from build123d import *

# Parameters (mm, degrees)
F0_R     = 12.5
F2_DEPTH = 10
F3_R     = 6.5
F4_DEPTH = 10
F1_R     = 6.5
F5_DEPTH = 10
F7_DEPTH = 10


with BuildPart() as f2:
    # F0 (on Top) → F2 (new body)
    with BuildSketch(Plane.XY):
        Circle(F0_R)
    extrude(amount=F2_DEPTH)

    # F3 (on Top) → F4 (join)
    with BuildSketch(Plane.XY):
        with BuildLine():
            Line((34.328218, 24.012301), (2.916428, 13.975679))
            Line((2.916428, 13.975679), (5.668561, 29.53591))
            ThreePointArc((5.668561, 29.53591), (7.450694, 29.144745), (9.261052, 28.917566))
            ThreePointArc((9.261052, 28.917566), (13.244302, 30.419157), (14.627135, 34.445176))
            ThreePointArc((14.627135, 34.445176), (8.904501, 45.49223), (-2.762528, 49.812691))
            ThreePointArc((-2.762528, 49.812691), (-2.862519, 49.810248), (-2.962442, 49.805804))
            ThreePointArc((-2.962442, 49.805804), (-9.528349, 46.776185), (-12.229052, 40.068284))
            Line((-12.229052, 40.068284), (-12.390435, 7.09241))
            Line((-12.390435, 7.09241), (-26.338638, 14.51822))
            ThreePointArc((-26.338638, 14.51822), (-25.415909, 16.092253), (-24.640417, 17.743804))
            ThreePointArc((-24.640417, 17.743804), (-24.837623, 21.996117), (-28.239276, 24.555377))
            ThreePointArc((-28.239276, 24.555377), (-40.51404, 22.526556), (-48.228353, 12.765648))
            ThreePointArc((-48.228353, 12.765648), (-48.256928, 12.669795), (-48.283579, 12.57339))
            ThreePointArc((-48.283579, 12.57339), (-47.431217, 5.392638), (-41.886188, 0.751261))
            Line((-41.886188, 0.751261), (-10.574138, -9.592329))
            Line((-10.574138, -9.592329), (-21.946735, -20.563157))
            ThreePointArc((-21.946735, -20.563157), (-23.158589, -19.199186), (-24.489668, -17.951293))
            ThreePointArc((-24.489668, -17.951293), (-28.594798, -16.824809), (-32.079968, -19.269118))
            ThreePointArc((-32.079968, -19.269118), (-33.943555, -31.570053), (-27.044233, -41.923087))
            ThreePointArc((-27.044233, -41.923087), (-26.961902, -41.979883), (-26.878451, -42.035021))
            ThreePointArc((-26.878451, -42.035021), (-19.785755, -43.443351), (-13.658035, -39.60398))
            Line((-13.658035, -39.60398), (5.855259, -13.020795))
            Line((5.855259, -13.020795), (12.77481, -27.22695))
            ThreePointArc((12.77481, -27.22695), (11.103113, -27.958002), (9.50497, -28.838313))
            ThreePointArc((9.50497, -28.838313), (7.165066, -32.394421), (8.412765, -36.464347))
            ThreePointArc((8.412765, -36.464347), (19.535769, -42.037922), (31.514097, -38.675541))
            ThreePointArc((31.514097, -38.675541), (31.593556, -38.61479), (31.671783, -38.552462))
            ThreePointArc((31.671783, -38.552462), (35.202948, -32.242106), (33.445058, -25.227866))
            Line((33.445058, -25.227866), (14.192887, 1.545035))
            Line((14.192887, 1.545035), (29.842002, 3.735976))
            ThreePointArc((29.842002, 3.735976), (30.020691, 1.920191), (30.364063, 0.128235))
            ThreePointArc((30.364063, 0.128235), (33.023052, -3.196044), (37.279343, -3.267088))
            ThreePointArc((37.279343, -3.267088), (46.017324, 5.589188), (46.521017, 18.020288))
            ThreePointArc((46.521017, 18.020288), (46.487793, 18.114631), (46.45269, 18.208289))
            ThreePointArc((46.45269, 18.208289), (41.542374, 23.516634), (34.328218, 24.012301))
        make_face()
        with Locations((-20.751796, -33.213474)):
            Circle(F3_R, mode=Mode.SUBTRACT)
        with Locations((25.175233, -29.999658)):
            Circle(F3_R, mode=Mode.SUBTRACT)
        with Locations((-38.000548, 9.472603)):
            Circle(F3_R, mode=Mode.SUBTRACT)
        with Locations((-2.733835, 39.067864)):
            Circle(F3_R, mode=Mode.SUBTRACT)
        with Locations((36.310946, 14.672665)):
            Circle(F3_R, mode=Mode.SUBTRACT)
    extrude(amount=F4_DEPTH)

    # F1 (on Top) → F5 (cut)
    with BuildSketch(Plane.XY):
        Circle(F1_R)
    extrude(amount=F5_DEPTH, mode=Mode.SUBTRACT)

    # F6 (on Top) → F7 (cut)
    with BuildSketch(Plane.XY):
        Polygon((0.315685, 27.979563), (-7.285573, 28.507008), (-7.38193, 8.817999), (-2.653955, 11.189572), align=None)
        Polygon((-26.512594, 8.946395), (-29.363142, 1.880158), (-10.667557, -4.295721), (-11.462033, 0.933707), align=None)
        Polygon((-16.701369, -22.450387), (-10.861847, -27.345007), (0.789017, -11.472901), (-4.429971, -10.61251), align=None)
        Polygon((16.19058, -22.821497), (22.650152, -18.780302), (11.155197, -2.794921), (8.72416, -7.492598), align=None)
        Polygon((26.707698, 8.345926), (24.86041, 15.738142), (6.105273, 9.745544), (9.821798, 5.981829), align=None)
    extrude(amount=F7_DEPTH, mode=Mode.SUBTRACT)


solid = f2.part
Design review of the part built by this model. Coordinates are the model's own, in mm. A direction names the side the tool comes from. Coordinates: 2 decimals unless noted, no trailing zeros. Put each result on its own line as item: value.
1) The part is to be moulded in two halves that separate along Y. For faces 1 (the face through (12.405, -15.05, 4.93)), 2 (the face through (-4.04, -26.5, 4.93)), 3 (the face through (3, 7, 0)), say which applies: released by +Y, released by -Y, zero draft, split by the parting line, or undercut.
Response values:
face 1: undercut
face 2: released by -Y
face 3: zero draft
2) Take a section at A-A, the plane z = 2.75. Count the separate pieces of the cut face and the enclosed holes in it, and give its area (3 significant figures).
Response values:
separate pieces: 1
enclosed holes: 11
area: 3,000 mm²
3) Insertion check: P1, Ø12, axis at x = -1.5, y = 3, coming from the +Z side; P2, Ø4, axis at x = 20, z = 6, coming from the -Y side; P3, Ø4, axis at x = -15.5, z = 8, coming from the +Y side; P4, Ø8, axis at x = 0, y = 0, coming from the -Z side. Each pin has a flat end and moves straight along its axis. Give the tip position at first contact, or say it passes through.
Response values:
P1: stops at z = 10
P2: stops at y = -42.12
P3: stops at y = 9.81
P4: passes through
4) Tool access review of faces 4 (the face through (9.957, -5.111, 4.93)), 5 (the face through (-26.45, -4.35, 4.93)): name each direction out of +Z, -Z, +X, -X, +Y, -Y from which nothing blocks a thin tool from reaching the whole face with its end or side.
Response values:
face 4: +Z, -Z
face 5: +Z, -Z, -X
5) Wall thickness on L1, parallel to X at y = -37, z = 7 (3 decimals); L2, parallel to Y at x = -22.5, z = 2.75; L3, parallel to X at y = -21.5, z = 7.5: over which ranges is each line inside the solid? List them lowest first. Write a range as from..to.
Response values:
L1: x = -31.713..-26.035, -15.469..-11.747, 8.92..33.198
L2: y = -43.56..-39.47, -26.95..-19.91, -5.65..-0.39, 6.81..12.47
L3: x = -33.15..-15.72, -6.57..-0.37, 9.99..15.55, 18.3..30.76
